```python
from build123d import *

# Parameters (mm, degrees)
SKETCH1_W           = 59.5
SKETCH1_H           = 5
BOSS_EXTRUDE1_DEPTH = 5
SKETCH2_W           = 49.5
SKETCH2_H           = 5
BOSS_EXTRUDE2_DEPTH = 5
SKETCH3_W           = 34
SKETCH3_H           = 5
BOSS_EXTRUDE3_DEPTH = 5


with BuildPart() as part:
    # Sketch1 → Boss-Extrude1 (new body)
    with BuildSketch(Plane.XY):
        with Locations((58.644042166, -123.5)):
            Rectangle(SKETCH1_W, SKETCH1_H)
    extrude(amount=BOSS_EXTRUDE1_DEPTH)

    # Sketch2 → Boss-Extrude2 (add)
    with BuildSketch(Plane.XY.offset(5)):
        with Locations((58.644042166, -123.5)):
            Rectangle(SKETCH2_W, SKETCH2_H)
    extrude(amount=BOSS_EXTRUDE2_DEPTH)

    # Sketch3 → Boss-Extrude3 (add)
    with BuildSketch(Plane(origin=(0, 0, 0), x_dir=(-1, 0, 0), z_dir=(0, 0, -1))):
        with Locations((-63.394042166, -123.5)):
            Rectangle(SKETCH3_W, SKETCH3_H)
    extrude(amount=BOSS_EXTRUDE3_DEPTH)


solid = part.part
```
CAD build for the part. Positions are in the model's coordinates, mm. A direction names the side the tool comes from. Coordinates: 2 decimals unless noted, no trailing zeros. Loops run counter-clockwise (first coordinate to the right, second up) from the corner with the lowest first, then second, coordinate; pieces in that order, holes last. Notation, with made-up numbers: (25.5, 60.25) - (70.5, 60.25) arc R13 ccw to (70.5, 68.25) - close; hole circle Ø2 at (22, 41). An arc over 180 degrees is marked (long way). Use CSV: the item, a comma, the result in double quotes. Start each with the question number.
Q1. Cut at C-C, the plane x = 45. List the corners of the cut face in (y, z), then the cut area to 3 significant figures.
Q2. Cut at A-A, the plane y = -123.9. List the corners of the cut face in (x, z), then the cut area to 3 significant figures.
Q3. 3-axis set-ups, long thin cutter, end or side, ignore diameter. For faces 1 (the flat face through (64, -123, -5)), 2 (the flat face through (46.394, -124, -2)), 3 (the flat face through (83.394, -124, 7)), 4 (the flat face through (80.394, -124, -2)), 5 (the flat face through (31, -123, 5)): which of +Z, -Z, +X, -X, +Y, -Y reach the whole face in a straight line?
Q4. Drop flat-ended pins along their axis: P1, Ø2, axis at x = 81.5, y = -122, coming from the -Z side; P2, Ø2.5, axis at y = -122.5, z = -3.5, coming from the -X side; P3, Ø3, axis at y = -123.5, z = -1, coming from the +X side; P4, Ø2.5, axis at y = -122.5, z = 8, coming from the +X side. Give the stop position or say it passes through.
Q5. Cut at B-B, the plane z = -2.5. List the corners of the cut face in (x, y), then the cut area to 3 significant figures.
Q6. Probe probe 1 along X at (y, z) = (-122.2, -3.5); probe 2 along X at (y, z) = (-125, 6.75); probe 3 along Z at (x, y) = (41, -123.8). List the from-to ranges inside material, lowest first. Write a range as from..to.
Here are the results:
1,outline,"(-126, 0) - (-121, 0) - (-121, 10) - (-126, 10) - close"
1,area,"50.0 mm2"
2,outline,"(28.89, 0) - (46.39, 0) - (46.39, -5) - (80.39, -5) - (80.39, 0) - (88.39, 0) - (88.39, 5) - (83.39, 5) - (83.39, 10) - (33.89, 10) - (33.89, 5) - (28.89, 5) - close"
2,area,"715 mm2"
3,face 1,"-Z, +X, -X, +Y, -Y"
3,face 2,"-Z, -X, +Y, -Y"
3,face 3,"+Z, +X, +Y, -Y"
3,face 4,"-Z, +X, +Y, -Y"
3,face 5,"+Z, -X, +Y, -Y"
4,P1,"z = 0"
4,P2,"x = 46.39"
4,P3,"x = 88.39"
4,P4,"x = 83.39"
5,outline,"(46.39, -126) - (80.39, -126) - (80.39, -121) - (46.39, -121) - close"
5,area,"170 mm2"
6,probe 1,"46.39..80.39"
6,probe 2,"33.89..83.39"
6,probe 3,"0..10"
